Source: CAD feature listing. Evaluate the final solid. Frame: model axes, mm. A direction names the side the tool comes from. Round coordinates to 2 decimals unless told otherwise and drop trailing zeros. Loops run counter-clockwise (first coordinate to the right, second up) from the corner with the lowest first, then second, coordinate; pieces in that order, holes last.
(1) Section B-B, the plane x = 21. Return the cut outline in (y, z), plus the area to 3 significant figures.
(2) Mould query, pull axis Z, two halves, no side actions, for faces 5 (the cylindrical face through (41.305, -11.513, 7.888)), 6 (the flat face through (29, -27, 16)), 7 (the flat face through (42, -28, 8)). Classes: pulls with the +Z half, pulls with the -Z half, needs draft (parallel to the pull), parting line crosses it, or undercut.
(3) First-contact query: pin 1 Ø4 at (x, y) = (41.5, -13) entering from +Z; pin 2 Ø6.5 at (y, z) = (-18.5, 8) entering from -X; pin 3 Ø8 at (y, z) = (-35.5, 10.5) entering from -X; pin 4 Ø8 at (x, z) = (6, 13.5) entering from -Y. Flat tips, straight axial feed; report the tip coordinate or a pass-through.
(4) Section D-D, the plane y = -16.5. Return the cut outline in (x, z), plus the area to 3 significant figures.
(5) Section C-C, the plane z = 14.75. Return the cut outline in (x, y), plus the area to 3 significant figures.
(6) Set-up query: faces 1 (the cylindrical face through (44.03, -36.11, 6.39)), 2 (the flat face through (18, -35, 8)), 3 (the flat face through (29, -27, 0)), 4 (the flat face through (26, -26, 8)). Return all of +Z, -Z, +X, -X, +Y, -Y with unobstructed straight access to the full face (end or side cutting, diameter ignored); none if empty.
(7) Section A-A, the plane z = 8. Return the cut outline in (x, y).
(8) Material intervals for probe 1 along Y at (x, z) = (24, 5.75); probe 2 along Y at (x, z) = (37.5, 7.75); probe 3 along X at (y, z) = (-13, 9.25), sorted ascending.
```python
from build123d import *

# Parameters (mm, degrees)
ESBO_O1_R                = 1.5
RESSALTO_EXTRUS_O1_DEPTH = 16
CHANFRO1_SIZE            = 2
ESBO_O2_R                = 5.5
CORTE_EXTRUS_O1_DEPTH    = 59.455110983
ESBO_O5_R                = 3
CORTE_EXTRUS_O2_DEPTH    = 16


with BuildPart() as part:
    # Esboço1 → Ressalto-extrusão1 (new body)
    with BuildSketch(Plane.XY):
        with BuildLine():
            Line((48, 0), (0, 0))
            Line((0, 0), (0, -11))
            Line((0, -11), (33.5, -11))
            ThreePointArc((33.5, -11), (35, -9.5), (36.5, -11))
            ThreePointArc((36.5, -11), (36.060660172, -12.060660172), (35, -12.5))
            Line((35, -12.5), (35, -24.5))
            ThreePointArc((35, -24.5), (36.060660172, -24.939339828), (36.5, -26))
            ThreePointArc((36.5, -26), (35, -27.5), (33.5, -26))
            Line((33.5, -26), (18, -26))
            Line((18, -26), (18, -44))
            Line((18, -44), (48, -44))
            Line((48, -44), (48, 0))
        make_face()
        with Locations((41.5, -13)):
            Circle(ESBO_O1_R, mode=Mode.SUBTRACT)
    extrude(amount=RESSALTO_EXTRUS_O1_DEPTH)

    # Chanfro1
    chanfro1_edges = [part.edges().sort_by_distance(p)[0] for p in [
        (48, 0, 8),
    ]]
    chamfer(chanfro1_edges, length=CHANFRO1_SIZE)

    # Esboço2 → Corte-extrusão1 (cut, through all)
    with BuildSketch(Plane.ZY.offset(-35)):
        with Locations((8, -18.5)):
            Circle(ESBO_O2_R)
    extrude(amount=-CORTE_EXTRUS_O1_DEPTH, mode=Mode.SUBTRACT)

    # Esboço5 → Corte-extrusão2 (cut)
    with BuildSketch(Plane.XZ.offset(44)):
        with Locations(Location((41.5, 8, 0), (0, 0, 270))):
            Circle(ESBO_O5_R)
    extrude(amount=-CORTE_EXTRUS_O2_DEPTH, mode=Mode.SUBTRACT)


solid = part.part
```
Output values:
1. outline: (-44, 0) - (-26, 0) - (-26, 16) - (-44, 16) - close; (-11, 0) - (0, 0) - (0, 16) - (-11, 16) - close
1. area: 464 mm2
2. face 5: needs draft
2. face 6: pulls with the +Z half
2. face 7: undercut
3. pin 1: stops at z = 16
3. pin 2: passes through
3. pin 3: stops at x = 18
3. pin 4: stops at y = -11
4. outline: (35, 0) - (48, 0) - (48, 2.88) - (35, 2.88) - close; (35, 13.12) - (48, 13.12) - (48, 16) - (35, 16) - close
4. area: 74.8 mm2
5. outline: (0, -11) - (33.5, -11) arc R1.5 cw (long way) to (35, -12.5) - (35, -24.5) arc R1.5 cw (long way) to (33.5, -26) - (18, -26) - (18, -44) - (48, -44) - (48, -2) - (46, 0) - (0, 0) - close; hole circle Ø3 at (41.5, -13)
5. area: 1,240 mm2
6. face 1: -Y
6. face 2: +Z, -Z, -X, -Y
6. face 3: -Z, +X, -X, +Y, -Y
6. face 4: +Z, -Z, -X
7. outline: (0, -11) - (33.5, -11) arc R1.5 cw (long way) to (35, -12.5) - (35, -13) - (40, -13) arc R1.5 cw to (43, -13) - (48, -13) - (48, -2) - (46, 0) - (0, 0) - close; (18, -44) - (38.5, -44) - (38.5, -28) - (44.5, -28) - (44.5, -44) - (48, -44) - (48, -24) - (35, -24) - (35, -24.5) arc R1.5 cw (long way) to (33.5, -26) - (18, -26) - close
8. probe 1: y = -44 to -26, -11 to 0
8. probe 2: y = -44 to -23.99, -13.01 to 0
8. probe 3: x = 35 to 40, 43 to 48
